Build history of the part. All positions in model axes, mm. A direction names the side the tool comes from. Coordinates: 2 decimals unless noted, no trailing zeros. Order: outer loops, then holes, each group sorted by start corner. A loop starts at its lowest first (then second) coordinate and runs counter-clockwise, first axis right, second up. Notation, with made-up numbers: (14.25, 47) - (61.25, 47) arc R8 ccw to (61.25, 54) - close; hole circle Ø11 at (-28.5, 68.5). An arc over 180 degrees is marked (long way). One line per item, written item: value.
from build123d import *

# Parameters (mm, degrees)
BOSS_EXTRUDE1_DEPTH = 1
SKETCH2_R           = 1
CUT_EXTRUDE1_DEPTH  = 2
BOSS_EXTRUDE3_DEPTH = 2


with BuildPart() as part:
    # Sketch1 → Boss-Extrude1 (new body)
    with BuildSketch(Plane.XY):
        with BuildLine():
            Line((-37.408874503, 0), (-36.935496874, -1.52115571))
            ThreePointArc((-36.935496874, -1.52115571), (-31.538206109, -9.097817453), (-22.7, -12))
            Line((-22.7, -12), (-20.8, -12))
            Line((-20.8, -12), (-20.8, 0))
            Line((-20.8, 0), (-2.848874503, 0))
            Line((-2.848874503, 0), (-2.848874503, 12.956751258))
            Line((-2.848874503, 12.956751258), (6.330544431, 12.956751258))
            Line((6.330544431, 12.956751258), (7.591125497, 12.956751258))
            Line((7.591125497, 12.956751258), (7.591125497, 13))
            ThreePointArc((7.591125497, 13), (3.929960262, 21.838834765), (-4.908874503, 25.5))
            Line((-4.908874503, 25.5), (-24.908874503, 25.5))
            ThreePointArc((-24.908874503, 25.5), (-33.747709268, 21.838834765), (-37.408874503, 13))
            Line((-37.408874503, 13), (-37.408874503, 0))
        make_face()
    extrude(amount=BOSS_EXTRUDE1_DEPTH)

    # Sketch2 → Cut-Extrude1 (cut, through all)
    with BuildSketch(Plane.XY.offset(1)):
        with Locations((-8.658874503, 10.5)):
            Circle(SKETCH2_R)
        with Locations((-23.658874503, 10.5)):
            Circle(SKETCH2_R)
        with Locations((-16.158874503, 5.5)):
            Circle(SKETCH2_R)
    extrude(amount=-CUT_EXTRUDE1_DEPTH, mode=Mode.SUBTRACT)

    # Sketch8 → Boss-Extrude3 (add)
    with BuildSketch(Plane.XY.offset(1)):
        with BuildLine():
            Line((-2.848874503, 12.956751258), (3.166072925, 12.956751258))
            Line((3.166072925, 12.956751258), (3.367034903, 18.000639192))
            ThreePointArc((3.367034903, 18.000639192), (2.849823018, 20.366659135), (1.243261137, 22.178982899))
            ThreePointArc((1.243261137, 22.178982899), (-1.693696517, 23.571902881), (-4.908874503, 24.05))
            Line((-4.908874503, 24.05), (-24.908874503, 24.05))
            ThreePointArc((-24.908874503, 24.05), (-32.722404435, 20.813529932), (-35.958874503, 13))
            Line((-35.958874503, 13), (-35.958874503, 1.543887245))
            ThreePointArc((-35.958874503, 1.543887245), (-35.832184971, 0.056041311), (-35.455764157, -1.388964962))
            Line((-35.455764157, -1.388964962), (-35.389408707, -1.576681154))
            ThreePointArc((-35.389408707, -1.576681154), (-30.47080344, -8.080025204), (-22.7, -10.55))
            Line((-22.7, -10.55), (-21.8, -10.55))
            Line((-21.8, -10.55), (-21.8, -4.322233026))
            ThreePointArc((-21.8, -4.322233026), (-27.267294325, -0.393232372), (-29.358874503, 6.006271182))
            Line((-29.358874503, 6.006271182), (-29.358874503, 10.202170558))
            ThreePointArc((-29.358874503, 10.202170558), (-28.131966709, 13.904649986), (-24.936824853, 16.141774295))
            ThreePointArc((-24.936824853, 16.141774295), (-15.555605997, 17.446766156), (-6.215886942, 15.87199031))
            ThreePointArc((-6.215886942, 15.87199031), (-4.096264622, 14.53396256), (-2.848874503, 12.359765022))
            Line((-2.848874503, 12.359765022), (-2.848874503, 12.956751258))
        make_face()
    extrude(amount=-BOSS_EXTRUDE3_DEPTH)


solid = part.part
1. Band-saw the part on B-B, the plane y = 7.5. Give the cut face in (x, z), and give its area (3 significant figures).
Values found:
outline: (-37.41, 0) - (-35.96, 0) - (-35.96, -1) - (-29.36, -1) - (-29.36, 0) - (-2.85, 0) - (-2.85, 1) - (-37.41, 1) - close
area: 41.2 mm2
2. Probe line 1 along Y through (x, z) = (-18, 0.85); line 2 along X through (y, z) = (7.5, -0.7); line 3 along Z through (x, y) = (-19.5, 14.5). List the from-to ranges inside material, lowest first.
Values found:
line 1: y = 0 to 25.5
line 2: x = -35.96 to -29.36
line 3: z = 0 to 1
3. 3-axis set-ups, long thin cutter, end or side, ignore diameter. For faces 1 (the face through (-27.21, -0.47, -0.49)), 2 (the face through (-35.836, 0.077, -0.493)), 3 (the face through (-22.3, -10.55, -0.5)), 4 (the face through (-4.12, 14.56, -0.49)), 5 (the face through (-21.8, -7.5, -0.5)): which of +Z, -Z, +X, -X, +Y, -Y reach the whole face in a straight line?
Values found:
face 1: -Z, +X
face 2: -Z, -X, -Y
face 3: -Z, +X, -X, -Y
face 4: -Z, -Y
face 5: -Z, +X, -Y
4. Two-plate mould, pull along X, no slides. Class faces 6 (the face through (-33.65, 21.935, 0.493)), 7 (the face through (-20.8, -6.1, 0.5)), 8 (the face through (-22.705, 10.8, 0.507)), 9 (the face through (-14.8, 24.05, -0.5)): pulls with the +X half, pulls with the -X half, needs draft (parallel to the pull), parting line crosses it, or undercut.
Values found:
face 6: pulls with the -X half
face 7: pulls with the +X half
face 8: undercut
face 9: needs draft
5. Band-saw the part on A-A, the plane z = 0.4. Give the cut face in (x, y), and give its area (3 significant figures).
Values found:
outline: (-37.41, 0) - (-36.94, -1.52) arc R14.91 ccw to (-22.7, -12) - (-20.8, -12) - (-20.8, 0) - (-2.85, 0) - (-2.85, 12.96) - (7.59, 12.96) - (7.59, 13) arc R12.5 ccw to (-4.91, 25.5) - (-24.91, 25.5) arc R12.5 ccw to (-37.41, 13) - close; hole circle Ø2 at (-23.66, 10.5); hole circle Ø2 at (-16.16, 5.5); hole circle Ø2 at (-8.66, 10.5)
area: 1,090 mm2
6. Band-saw the part on C-C, the plane x = -33. Give the cut face in (y, z), and give its area (3 significant figures).
Values found:
outline: (-7.87, 0) - (-5.75, 0) - (-5.75, -1) - (20.53, -1) - (20.53, 0) - (22.53, 0) - (22.53, 1) - (-7.87, 1) - close
area: 56.7 mm2
7. Flat gauge pins, fed straight in: P1, Ø2, axis at x = -7, y = 10.5, coming from the -Z side; P2, Ø0.8, axis at x = -13.5, z = -0.5, coming from the +Y side; P3, Ø0.6, axis at x = 0, z = 0, coming from the -Y side. Where does each tip first touch, or does it go through?
Values found:
P1: stops at z = 0
P2: stops at y = 24.05
P3: stops at y = 12.96
